Could you check a few things on this model? Use its own coordinates, in mm. Face numbers are marked on the shaded views. Round coordinates to 2 decimals unless told otherwise and drop trailing zeros. Loops run counter-clockwise (first coordinate to the right, second up) from the corner with the lowest first, then second, coordinate; pieces in that order, holes last. Notation, with made-up numbers: (54, -40) -> (79, -40) arc R26 cw to (79, -14) -> close; hole circle Ø5 at (-2, 12.25). An arc over 180 degrees is marked (long way). Write each question's results on one line, items separated by ' | '.
from build123d import *

# Parameters (mm, degrees)
SKETCH002_W             = 85
SKETCH002_H             = 118
PAD001_DEPTH            = 38
THICKNESS001_T          = 1
SKETCH008_R             = 3.875
SKETCH008_R_2           = 5.9
POCKET_DEPTH            = 5
BODY001_PLACEMENT_ANGLE = 180


with BuildPart() as part:
    # Sketch002 → Pad001 (new body)
    with BuildSketch(Plane.XY):
        with Locations((42.5, 59)):
            Rectangle(SKETCH002_W, SKETCH002_H)
    extrude(amount=PAD001_DEPTH)

    # Thickness001
    thickness001_openings = [part.faces().sort_by_distance(p)[0] for p in [
        (85, 59, 19),
        (42.5, 59, 0),
        (0, 59, 19),
    ]]
    offset(amount=THICKNESS001_T, openings=thickness001_openings)

    # Sketch008 (on Face10 of Thickness001) → Pocket (cut)
    with BuildSketch(Plane.XZ.offset(1)):
        with Locations((63.75, 19)):
            Circle(SKETCH008_R)
        with Locations((21.25, 19)):
            Circle(SKETCH008_R)
        with Locations((42.5, 19)):
            Circle(SKETCH008_R_2)
    extrude(amount=-POCKET_DEPTH, mode=Mode.SUBTRACT)


with BuildPart() as part_1:
    # Body001 placement: moved
    add(part.part.moved(Location((0, 120, 0))).rotate(Axis((0, 120, 0), (1, 0, 0)), BODY001_PLACEMENT_ANGLE))


solid = part_1.part
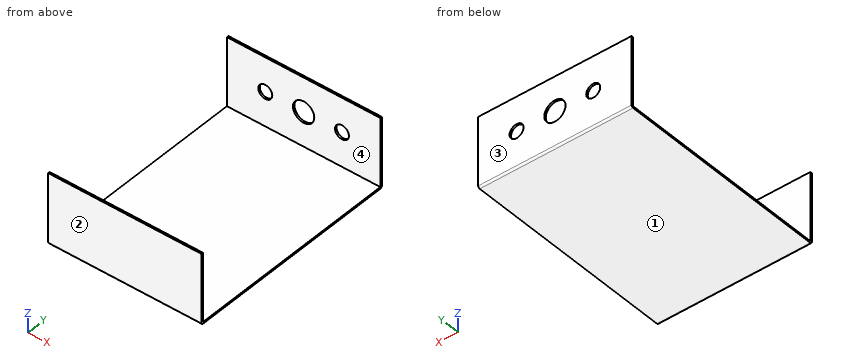
1) I want a section at C-C, the plane z = -19. Write out the boundary of the cut face in (x, y) (3 decimals), plus the area to 3 significant figures.
Model answer:
outline: (0, 1) -> (85, 1) -> (85, 2) -> (0, 2) -> close; (0, 120) -> (17.375, 120) -> (17.375, 121) -> (0, 121) -> close; (25.125, 120) -> (36.6, 120) -> (36.6, 121) -> (25.125, 121) -> close; (48.4, 120) -> (59.875, 120) -> (59.875, 121) -> (48.4, 121) -> close; (67.625, 120) -> (85, 120) -> (85, 121) -> (67.625, 121) -> close | area: 143 mm2
2) I need wall thicknesses on line 1 (X direction, y = 120.25, z = -19) (3 decimals); line 2 (Y direction, x = 26, z = -18); line 3 (Z direction, x = 63.75, y = 120.3) (3 decimals). Which ranges of each line are inside material? Lowest first, please.
Model answer:
line 1: x = 0 to 17.375, 25.125 to 36.6, 48.4 to 59.875, 67.625 to 85 | line 2: y = 1 to 2, 120 to 121 | line 3: z = -38.954 to -22.875, -15.125 to 0
3) If we mould it in two halves opening along Y, with no side actions, what happens to the marked faces 1, 2, 3 and 4? For each: released by +Y, released by -Y, zero draft, split by the parting line, or undercut.
Model answer:
face 1: zero draft | face 2: released by -Y | face 3: released by +Y | face 4: undercut
4) I want a section at D-D, the plane x = 42.5. Write out the boundary of the cut face in (y, z).
Model answer:
outline: (1, -38) arc R1 ccw to (2, -39) -> (120, -39) arc R1 ccw to (121, -38) -> (121, -24.9) -> (120, -24.9) -> (120, -38) -> (2, -38) -> (2, 0) -> (1, 0) -> close; (120, -13.1) -> (121, -13.1) -> (121, 0) -> (120, 0) -> close
5) I want a section at B-B, the plane z = -32. Write out the boundary of the cut face in (x, y).
Model answer:
outline: (0, 1) -> (85, 1) -> (85, 2) -> (0, 2) -> close; (0, 120) -> (85, 120) -> (85, 121) -> (0, 121) -> close
6) I'm going to push a flat-ended pin straight in: pin 1 (5 mm diameter, centred on x = 75.5, y = 13.5, fed in from +Z). Where does the tip first touch, or does it pass through?
Model answer:
pin 1: stops at z = -38
7) I want a section at A-A, the plane x = 21.25. Write out the boundary of the cut face in (y, z) (3 decimals).
Model answer:
outline: (1, -38) arc R1 ccw to (2, -39) -> (120, -39) arc R1 ccw to (121, -38) -> (121, -22.875) -> (120, -22.875) -> (120, -38) -> (2, -38) -> (2, 0) -> (1, 0) -> close; (120, -15.125) -> (121, -15.125) -> (121, 0) -> (120, 0) -> close
